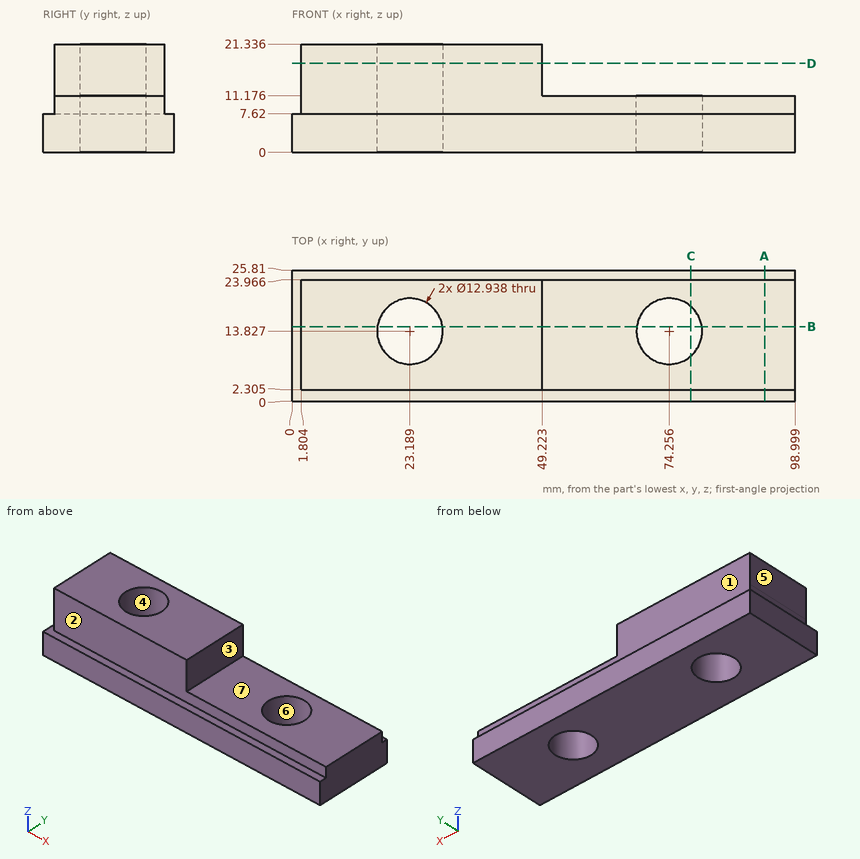
Job drawing, mm, ordinate dimensions from the low corner. One solid piece. A direction names the side the tool comes from. Coordinates: 2 decimals unless noted, no trailing zeros. Order: outer loops, then holes, each group sorted by start corner. A loop starts at its lowest first (then second) coordinate and runs counter-clockwise, first axis right, second up. Notation, with made-up numbers: (-11, 14.5) - (37, 14.5) arc R11 cw to (37, 27.5) - close; hole circle Ø5 at (-36, -13). An arc over 180 degrees is marked (long way). Return JSON: item names as keys, results as strings. Group by question number.
1) Saw through at C-C, the plane x = 78.5. Write the cut outline in (y, z) (1 decimal).
2) Saw through at D-D, the plane z = 17.5. Write the cut outline in (x, y) (1 decimal), plus the area to 3 significant figures.
3) Probe line 1 (X direction, y = 14.75, z = 1); line 2 (X direction, y = 11.75, z = 9.5) (1 decimal); line 3 (Z direction, x = 95, y = 4.75). List the from-to ranges inside material, lowest first. Write a range as from..to.
4) Mould opens along X. For the marked faces 4, 5, 6 and 7 say: released by +X, released by -X, zero draft, split by the parting line, or undercut.
5) Saw through at A-A, the plane x = 93. Write the cut outline in (y, z) (1 decimal), plus the area to 3 significant figures.
6) Saw through at B-B, the plane y = 14.75. Write the cut outline in (x, z) (1 decimal), plus the area to 3 significant figures.
7) Tool access for the marked faces 1, 2 and 3: list every direction of +Z, -Z, +X, -X, +Y, -Y with a clear straight run to the whole face (end or side of a thin tool).
8) Flat gauge pins, fed straight in: P1, Ø5, axis at y = 15.5, z = 17.5, coming from the +X side; P2, Ø4, axis at y = 16, z = 10.5, coming from the -X side; P3, Ø5, axis at x = 30, z = 17, coming from the +Y side. Where does each tip first touch, or does it go through?
Values found:
{
 "1": {"outline": "(0, 0) - (8.9, 0) - (8.9, 11.2) - (2.3, 11.2) - (2.3, 7.6) - (0, 7.6) - close; (18.7, 0) - (25.8, 0) - (25.8, 7.6) - (24, 7.6) - (24, 11.2) - (18.7, 11.2) - close"},
 "2": {"outline": "(1.8, 2.3) - (49.2, 2.3) - (49.2, 24) - (1.8, 24) - close; hole circle Ø12.9 at (23.2, 13.8)", "area": "896 mm²"},
 "3": {"line 1": "x = 0..16.79, 29.59..67.85, 80.66..99", "line 2": "x = 1.8..17.1, 29.3..68.1, 80.4..99", "line 3": "z = 0..11.18"},
 "4": {"face 4": "undercut", "face 5": "released by -X", "face 6": "undercut", "face 7": "zero draft"},
 "5": {"outline": "(0, 0) - (25.8, 0) - (25.8, 7.6) - (24, 7.6) - (24, 11.2) - (2.3, 11.2) - (2.3, 7.6) - (0, 7.6) - close", "area": "274 mm²"},
 "6": {"outline": "(0, 0) - (16.8, 0) - (16.8, 21.3) - (1.8, 21.3) - (1.8, 7.6) - (0, 7.6) - close; (29.6, 0) - (67.9, 0) - (67.9, 11.2) - (49.2, 11.2) - (49.2, 21.3) - (29.6, 21.3) - close; (80.7, 0) - (99, 0) - (99, 11.2) - (80.7, 11.2) - close", "area": "1,170 mm²"},
 "7": {"face 1": "+Z, +X, -X, +Y", "face 2": "+Z, +X, -X, -Y", "face 3": "+Z, +X, +Y, -Y"},
 "8": {"P1": "stops at x = 49.22", "P2": "stops at x = 1.8", "P3": "stops at y = 23.97"}
}
